```python
from build123d import *

# Parameters (mm, degrees)
SKETCH1_R           = 84.7725
SKETCH1_R_2         = 6.35
BOSS_EXTRUDE1_DEPTH = 6.35
SKETCH4_R           = 14.2875
CUT_EXTRUDE1_DEPTH  = 9.652


with BuildPart() as part:
    # Sketch1 → Boss-Extrude1 (new body)
    with BuildSketch(Plane(origin=(0, 0, 0), x_dir=(1, 0, 0), z_dir=(0, 1, 0))):
        with BuildLine():
            Line((273.05, 114.3), (-95.25, 114.3))
            ThreePointArc((-95.25, 114.3), (-99.740128061, 112.440128061), (-101.6, 107.95))
            Line((-101.6, 107.95), (-101.6, -95.25))
            ThreePointArc((-101.6, -95.25), (-99.740128061, -99.740128061), (-95.25, -101.6))
            Line((-95.25, -101.6), (241.3, -101.6))
            ThreePointArc((241.3, -101.6), (245.790128061, -99.740128061), (247.65, -95.25))
            Line((247.65, -95.25), (247.65, -12.7))
            ThreePointArc((247.65, -12.7), (249.509871939, -8.209871939), (254, -6.35))
            Line((254, -6.35), (273.05, -6.35))
            ThreePointArc((273.05, -6.35), (277.540128061, -4.490128061), (279.4, 0))
            Line((279.4, 0), (279.4, 107.95))
            ThreePointArc((279.4, 107.95), (277.540128061, 112.440128061), (273.05, 114.3))
        make_face()
        with Locations(Location((0, 0, 0), (0, 0, 270))):
            Circle(SKETCH1_R, mode=Mode.SUBTRACT)
        with Locations(Location((-90.060644326, -31.010366712, 0), (0, 0, 270))):
            Circle(SKETCH1_R_2, mode=Mode.SUBTRACT)
        with Locations(Location((18.17455681, 93.499989223, 0), (0, 0, 270))):
            Circle(SKETCH1_R_2, mode=Mode.SUBTRACT)
        with Locations(Location((71.886087516, -62.489622511, 0), (0, 0, 270))):
            Circle(SKETCH1_R_2, mode=Mode.SUBTRACT)
        with Locations(Location((266.7, 88.9, 0), (0, 0, 270))):
            Circle(SKETCH1_R_2, mode=Mode.SUBTRACT)
        with Locations(Location((266.7, 25.4, 0), (0, 0, 270))):
            Circle(SKETCH1_R_2, mode=Mode.SUBTRACT)
    extrude(amount=BOSS_EXTRUDE1_DEPTH)

    # Sketch4 → Cut-Extrude1 (cut)
    with BuildSketch(Plane(origin=(0, 6.35, 0), x_dir=(1, 0, 0), z_dir=(0, 1, 0))):
        with Locations(Location((195.68668, -50.292, 0), (0, 0, 270))):
            Circle(SKETCH4_R)
    extrude(amount=-CUT_EXTRUDE1_DEPTH, mode=Mode.SUBTRACT)


solid = part.part
```
Work out the finished part from the listing and answer in its coordinate system (mm). Round coordinates to 2 decimals unless told otherwise and drop trailing zeros. Write each loop counter-clockwise with the first axis right and the second up, starting at its lowest first coordinate (ties: lowest second). Pieces come first, ordered by that corner, then holes. Notation, with made-up numbers: (72, 73) - (125, 73) arc R17 cw to (125, 101) - close; hole circle Ø4 at (69.5, 75.5). An arc over 180 degrees is marked (long way). Return JSON: item names as keys, results as strings. Group by question number.
Q1. The mould has two halves that part along Z. Classify faces 1 (the cylindrical face through (260.5, 3.13, -26.78)), 2 (the flat face through (129, 6.35, -8)): released by +Z, released by -Z, zero draft, split by the parting line, or undercut.
Q2. Find the intervals of material crossed by L1, parallel to Z at x = 266.7, y = 2.5; L2, parallel to X at y = 6.25, z = -1; L3, parallel to X at y = 2, z = 59, in increasing order.
Q3. The part is cut by section C-C on z = -6.5. Write down the section's boundary in (x, y), then the cut area to 3 significant figures.
Q4. The part is cut by section B-B on x = 0. Write down the section's boundary in (y, z), then the cut area to 3 significant figures.
Q5. The part is cut by section A-A on x = 266.7. Write down the section's boundary in (y, z), then the cut area to 3 significant figures.
Q6. The part is cut by section D-D on y = 5. Count the separate pieces of the cut face and the enclosed holes in it, then the cut area to 3 significant figures.
Q7. Each of these flat-tipped pins is pushed along its axis until it touches: pin 1 Ø1.9 at (y, z) = (3, 42.5) entering from +X; pin 2 Ø23 at (x, z) = (195.69, 50.29) entering from -Y; pin 3 Ø1.9 at (x, y) = (266.5, 4) entering from +Z. Where does it stop, or does it pass through?
Solved:
{
 "1": {"face 1": "undercut", "face 2": "zero draft"},
 "2": {"L1": "-114.3 to -95.25, -82.55 to -31.75, -19.05 to 6.35", "L2": "-101.6 to -84.77, 84.77 to 279.4", "L3": "-101.6 to -60.87, 60.87 to 66.58, 77.19 to 184.36, 207.01 to 247.65"},
 "3": {"outline": "(-101.6, 0) - (-84.52, 0) - (-84.52, 6.35) - (-101.6, 6.35) - close; (84.52, 0) - (279.4, 0) - (279.4, 6.35) - (84.52, 6.35) - close", "area": "1,350 mm²"},
 "4": {"outline": "(0, -114.3) - (6.35, -114.3) - (6.35, -84.77) - (0, -84.77) - close; (0, 84.77) - (6.35, 84.77) - (6.35, 101.6) - (0, 101.6) - close", "area": "294 mm²"},
 "5": {"outline": "(0, -114.3) - (6.35, -114.3) - (6.35, -95.25) - (0, -95.25) - close; (0, -82.55) - (6.35, -82.55) - (6.35, -31.75) - (0, -31.75) - close; (0, -19.05) - (6.35, -19.05) - (6.35, 6.35) - (0, 6.35) - close", "area": "605 mm²"},
 "6": {"separate pieces": "1", "enclosed holes": "7", "area": "55,300 mm²"},
 "7": {"pin 1": "x = 247.65", "pin 2": "through", "pin 3": "z = 6.35"}
}
